from build123d import *

# Parameters (mm, degrees)
SKETCH_1_R          = 30
EXTRUDE_1_DEPTH     = 35
SKETCH_2_R          = 1.65
CUT_EXTRUDE_1_DEPTH = 56
SKETCH_4_R          = 20
CUT_EXTRUDE_3_DEPTH = 10
SKETCH_5_R          = 4
CUT_EXTRUDE_4_DEPTH = 50.244289009
SKETCH_6_R          = 2.15
CUT_EXTRUDE_5_DEPTH = 50.244289009


with BuildPart() as part:
    # 草图1 → 凸台-拉伸1 (new body)
    with BuildSketch(Plane(origin=(0, 0, 0), x_dir=(1, 0, 0), z_dir=(0, 1, 0))):
        with Locations(Location((0, 0, 0), (0, 0, 270))):
            Circle(SKETCH_1_R)
    extrude(amount=EXTRUDE_1_DEPTH)

    # 草图2 → 切除-拉伸1 (cut, through all)
    with BuildSketch(Plane.XZ):
        with Locations(Location((-26.25, 0, 0), (0, 0, 270))):
            Circle(SKETCH_2_R)
        with Locations(Location((-20.108666632, 16.873174754, 0), (0, 0, 270))):
            Circle(SKETCH_2_R)
        with Locations(Location((-4.558264664, 25.851203517, 0), (0, 0, 270))):
            Circle(SKETCH_2_R)
        with Locations(Location((13.125, 22.733166849, 0), (0, 0, 270))):
            Circle(SKETCH_2_R)
        with Locations(Location((24.666931296, 8.978028762, 0), (0, 0, 270))):
            Circle(SKETCH_2_R)
        with Locations(Location((24.666931296, -8.978028762, 0), (0, 0, 270))):
            Circle(SKETCH_2_R)
        with Locations(Location((13.125, -22.733166849, 0), (0, 0, 270))):
            Circle(SKETCH_2_R)
        with Locations(Location((-4.558264664, -25.851203517, 0), (0, 0, 270))):
            Circle(SKETCH_2_R)
        with Locations(Location((-20.108666632, -16.873174754, 0), (0, 0, 270))):
            Circle(SKETCH_2_R)
    extrude(amount=-CUT_EXTRUDE_1_DEPTH, mode=Mode.SUBTRACT)

    # 草图4 → 切除-拉伸3 (cut)
    with BuildSketch(Plane.XZ):
        with Locations(Location((0, 0, 0), (0, 0, 270))):
            Circle(SKETCH_4_R)
    extrude(amount=-CUT_EXTRUDE_3_DEPTH, mode=Mode.SUBTRACT)

    # 草图5 → 切除-拉伸4 (cut, through all)
    with BuildSketch(Plane.XZ.offset(-10)):
        with Locations(Location((0, 0, 0), (0, 0, 270))):
            Circle(SKETCH_5_R)
    extrude(amount=-CUT_EXTRUDE_4_DEPTH, mode=Mode.SUBTRACT)

    # 草图6 → 切除-拉伸5 (cut, through all)
    with BuildSketch(Plane.XZ.offset(-10)):
        with Locations(Location((0, 12, 0), (0, 0, 270))):
            Circle(SKETCH_6_R)
        with Locations(Location((12, 0, 0), (0, 0, 270))):
            Circle(SKETCH_6_R)
        with Locations(Location((0, -12, 0), (0, 0, 270))):
            Circle(SKETCH_6_R)
        with Locations(Location((-12, 0, 0), (0, 0, 270))):
            Circle(SKETCH_6_R)
    extrude(amount=-CUT_EXTRUDE_5_DEPTH, mode=Mode.SUBTRACT)


solid = part.part
Check sheet for the modelled part. Datum: model origin and axes. Units: mm. A direction names the side the tool comes from. Give positions to 0.01 mm unless a question says otherwise; leave off trailing zeros. Loops run counter-clockwise (first coordinate to the right, second up) from the corner with the lowest first, then second, coordinate; pieces in that order, holes last. Notation, with made-up numbers: M -37.5,77.5 L 1.5,77.5 A14 cw 1.5,96.5 Z; hole C 14,-36.75 d10. An arc over 180 degrees is marked long. Use a Markdown table: item, result. Add a question column.
Q1. Sectioned sample at D-D, the plane x = 25.5. Record the cut outline in (y, z), then the cut area to 3 significant figures.
Q2. Sectioned sample at C-C, the plane z = 22. Record the cut outline in (x, y), then the cut area to 3 significant figures.
Q3. Sectioned sample at A-A, the plane z = 0. Record the cut outline in (x, y), then the cut area to 3 significant figures.
Q4. Sectioned sample at B-B, the plane x = 0. Record the cut outline in (y, z), then the cut area to 4 significant figures.
Q5. Go/stop test with flat-tipped pins: pin 1 (4 mm diameter, centred on y = 19.5, z = 4, fed in from +X); pin 2 (1.5 mm diameter, centred on x = 8, z = 16, fed in from -Y); pin 3 (1 mm diameter, centred on y = 14, z = 0, fed in from -X). Record where each tip stops, or that it passes through.
Q6. Tool access check on faces 5 (the cylindrical face through (-5.56, 17.26, -24.54)), 6 (the flat face through (-4.2, 10, 0.3)). Record the directions out of +Z, -Z, +X, -X, +Y, -Y that give a thin tool (end or side, any length) a straight path to the whole face; none if there is none.
Q7. Mould release check, pull along Z, two halves, no side actions. Record for faces 1 (the cylindrical face through (25.782, 17.255, 10.194)), 2 (the cylindrical face through (1.32, 17.26, -29.97)), 3 (the flat face through (-6, 0, 20)), 4 (the cylindrical face through (0.65, 22.32, 9.95)): pulls with the +Z half, pulls with the -Z half, needs draft (parallel to the pull), parting line crosses it, or undercut.
Q8. Scan lines: line 1 along X through (y, z) = (23, 0); line 2 along Z through (x, y) = (-0.5, 3.5); line 3 along X through (y, z) = (27, 12). Record each from-to range of solid material in increasing order. Write a range as [from, to].
Verdict:
| question | item | result |
|---|---|---|
| 1 | outline | M 0,-15.8 L 35,-15.8 L 35,-10.4 L 0,-10.4 Z; M 0,-7.55 L 35,-7.55 L 35,7.55 L 0,7.55 Z; M 0,10.4 L 35,10.4 L 35,15.8 L 0,15.8 Z |
| 1 | area | 907 mm^2 |
| 2 | outline | M -20.4,0 L 11.65,0 L 11.65,35 L -20.4,35 Z; M 14.6,0 L 20.4,0 L 20.4,35 L 14.6,35 Z |
| 2 | area | 1,320 mm^2 |
| 3 | outline | M -30,0 L -27.9,0 L -27.9,35 L -30,35 Z; M -24.6,0 L -20,0 L -20,10 L -14.15,10 L -14.15,35 L -24.6,35 Z; M -9.85,10 L -4,10 L -4,35 L -9.85,35 Z; M 4,10 L 9.85,10 L 9.85,35 L 4,35 Z; M 14.15,10 L 20,10 L 20,0 L 30,0 L 30,35 L 14.15,35 Z |
| 3 | area | 1,170 mm^2 |
| 4 | outline | M 0,-30 L 35,-30 L 35,-14.15 L 10,-14.15 L 10,-20 L 0,-20 Z; M 0,20 L 10,20 L 10,14.15 L 35,14.15 L 35,30 L 0,30 Z; M 10,-9.85 L 35,-9.85 L 35,-4 L 10,-4 Z; M 10,4 L 35,4 L 35,9.85 L 10,9.85 Z |
| 4 | area | 1,285 mm^2 |
| 5 | pin 1 | x = 29.93 |
| 5 | pin 2 | y = 10 |
| 5 | pin 3 | x = -30 |
| 6 | face 5 | +Y, -Y |
| 6 | face 6 | -Y |
| 7 | face 1 | undercut |
| 7 | face 2 | parting line crosses it |
| 7 | face 3 | needs draft |
| 7 | face 4 | undercut |
| 8 | line 1 | [-30, -27.9], [-24.6, -14.15], [-9.85, -4], [4, 9.85], [14.15, 30] |
| 8 | line 2 | [-30, -19.99], [19.99, 30] |
| 8 | line 3 | [-27.5, -2.15], [2.15, 27.5] |
